Read the model definition and answer for the solid it produces. Units are mm, in the model's axes. Coordinates: 2 decimals unless noted, no trailing zeros. Loops run counter-clockwise (first coordinate to the right, second up) from the corner with the lowest first, then second, coordinate; pieces in that order, holes last. Notation, with made-up numbers: M 30,3.5 L 59,3.5 A25 ccw 59,42.5 Z; hole C 28.25,40 d6. An arc over 180 degrees is marked long. Use one line per item in the form item = value. Start each with the question number.
1. The part is cut by section C-C (x = -56). Give the vertices of the cut face in (y, z).
2. The part is cut by section A-A (x = -100). Give the vertices of the cut face in (y, z), plus the area to 3 significant figures.
3. A flat-ended cylindrical pin translates along its axis: pin 1 (10 mm diameter, centred on x = -56, y = 7.5, fed in from +Z). Find the tip coordinate at first contact, or state that the pin passes through.
4. Find the intervals of material crossed by probe 1 along Y at (x, z) = (78, 0.75); probe 2 along X at (y, z) = (7.5, 1.6); probe 3 along Y at (x, z) = (77, 0.5), in increasing order. Write a range as [from, to].
5. The part is cut by section B-B (y = -59). Give the vertices of the cut face in (x, z).
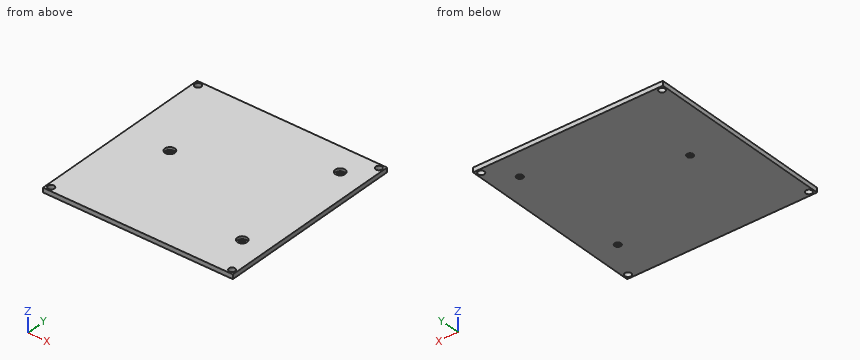
from build123d import *

# Parameters (mm, degrees)
F0_W     = 210
F0_H     = 210
F0_R     = 3.5
F1_DEPTH = 5
F2_R     = 5.5
F3_DEPTH = 3


with BuildPart() as f1:
    # F0 (on Top) → F1 (new body)
    with BuildSketch(Plane.XY):
        Rectangle(F0_W, F0_H)
        with Locations((-100, -100)):
            Circle(F0_R, mode=Mode.SUBTRACT)
        with Locations((100, -100)):
            Circle(F0_R, mode=Mode.SUBTRACT)
        with Locations((78, -59)):
            Circle(F0_R, mode=Mode.SUBTRACT)
        with Locations((-56, 7.5)):
            Circle(F0_R, mode=Mode.SUBTRACT)
        with Locations((-100, 100)):
            Circle(F0_R, mode=Mode.SUBTRACT)
        with Locations((78, 74.5)):
            Circle(F0_R, mode=Mode.SUBTRACT)
        with Locations((100, 100)):
            Circle(F0_R, mode=Mode.SUBTRACT)
    extrude(amount=F1_DEPTH)

    # F2 (on face) → F3 (cut)
    with BuildSketch(Plane.XY.offset(5)):
        with Locations((-56, 7.5)):
            Circle(F2_R)
        with Locations((78, 74.5)):
            Circle(F2_R)
        with Locations((78, -59)):
            Circle(F2_R)
    extrude(amount=-F3_DEPTH, mode=Mode.SUBTRACT)


solid = f1.part
Computed values:
q1.outline = M -105,0 L 4,0 L 4,2 L 2,2 L 2,5 L -105,5 Z; M 11,0 L 105,0 L 105,5 L 13,5 L 13,2 L 11,2 Z
q2.outline = M -105,0 L -103.5,0 L -103.5,5 L -105,5 Z; M -96.5,0 L 96.5,0 L 96.5,5 L -96.5,5 Z; M 103.5,0 L 105,0 L 105,5 L 103.5,5 Z
q2.area = 980 mm²
q3.pin_1 = 2
q4.probe_1 = [-105, -62.5], [-55.5, 71], [78, 105]
q4.probe_2 = [-105, -59.5], [-52.5, 105]
q4.probe_3 = [-105, -62.35], [-55.65, 71.15], [77.85, 105]
q5.outline = M -105,0 L 74.5,0 L 74.5,2 L 72.5,2 L 72.5,5 L -105,5 Z; M 81.5,0 L 105,0 L 105,5 L 83.5,5 L 83.5,2 L 81.5,2 Z
